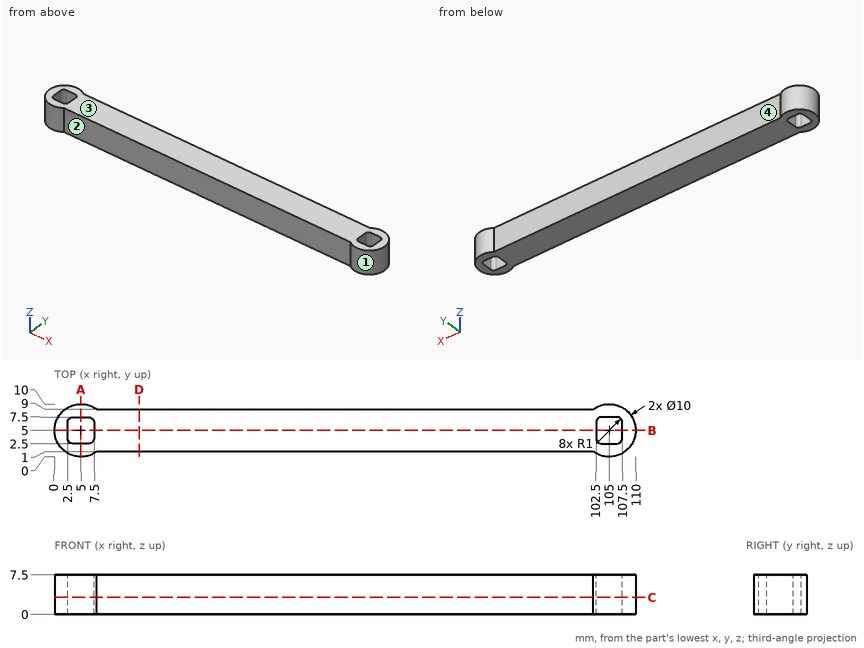
Job drawing, mm, ordinate dimensions from the low corner. One solid piece. Round coordinates to 2 decimals unless told otherwise and drop trailing zeros. Loops run counter-clockwise (first coordinate to the right, second up) from the corner with the lowest first, then second, coordinate; pieces in that order, holes last.
Item 1: Cut at C-C, the plane z = 3.25. Give the cut face in (x, y), then the cut area to 3 significant figures.
Item 2: Cut at A-A, the plane x = 5. Give the cut face in (y, z), then the cut area to 3 significant figures.
Item 3: Mould opens along Y. For the marked faces 1, 2, 3 and 4 say: +Y half, -Y half, draft (parallel to the pull), parting line (faces both ways), or undercut.
Item 4: Cut at D-D, the plane x = 16. Give the cut face in (y, z).
Item 5: Drop flat-ended pins along their axis: P1, Ø2, axis at x = 78, z = 3, coming from the -Y side; P2, Ø2, axis at y = 9, z = 2, coming from the -X side; P3, Ø1.5, axis at y = 6.5, z = 6, coming from the -X side. Give the stop position or say it passes through.
Item 6: Cut at B-B, the plane y = 5. Give the cut face in (x, z).
Item 7: Drill centre lines: line 1 (X direction, y = 5.25, z = 1.75); line 2 (X direction, y = 3, z = 1.25); line 3 (Y direction, x = 67, z = 4.5). Where is each one in solid material? Low to high.
A:
1. outline: (8, 1) - (102, 1) arc R5 ccw (long way) to (102, 9) - (8, 9) arc R5 ccw (long way) to start; hole (2.5, 3.5) arc R1 ccw to (3.5, 2.5) - (6.5, 2.5) arc R1 ccw to (7.5, 3.5) - (7.5, 6.5) arc R1 ccw to (6.5, 7.5) - (3.5, 7.5) arc R1 ccw to (2.5, 6.5) - close; hole (102.5, 3.5) arc R1 ccw to (103.5, 2.5) - (106.5, 2.5) arc R1 ccw to (107.5, 3.5) - (107.5, 6.5) arc R1 ccw to (106.5, 7.5) - (103.5, 7.5) arc R1 ccw to (102.5, 6.5) - close
1. area: 838 mm2
2. outline: (0, 0) - (2.5, 0) - (2.5, 7.5) - (0, 7.5) - close; (7.5, 0) - (10, 0) - (10, 7.5) - (7.5, 7.5) - close
2. area: 37.5 mm2
3. face 1: parting line
3. face 2: -Y half
3. face 3: draft
3. face 4: +Y half
4. outline: (1, 0) - (9, 0) - (9, 7.5) - (1, 7.5) - close
5. P1: stops at y = 1
5. P2: stops at x = 1
5. P3: stops at x = 0.06
6. outline: (0, 0) - (2.5, 0) - (2.5, 7.5) - (0, 7.5) - close; (7.5, 0) - (102.5, 0) - (102.5, 7.5) - (7.5, 7.5) - close; (107.5, 0) - (110, 0) - (110, 7.5) - (107.5, 7.5) - close
7. line 1: x = 0.01 to 2.5, 7.5 to 102.5, 107.5 to 109.99
7. line 2: x = 0.42 to 2.63, 7.37 to 102.63, 107.37 to 109.58
7. line 3: y = 1 to 9
